```python
from build123d import *

# Parameters (mm, degrees)
F0_W         = 50.8
F0_H         = 25.4
F0_R         = 3.3655
F1_DEPTH     = 17.78
F2_W         = 9.906
F2_H         = 25.4
F3_DEPTH     = 9.906
F5_DEPTH     = 2.54
F6_R         = 5.08
F7_T1_DEPTH  = 25.4
F7_T3_DEPTH  = 4.826
F7_T5_DEPTH  = 15.24
F7_T7_DEPTH  = 2.286
F7_T10_ANGLE = 90
F7_T12_ANGLE = 90
F7_T14_ANGLE = 90
F7_T16_ANGLE = 90
F7_T18_ANGLE = 90
F7_T20_ANGLE = 90
F7_T22_ANGLE = 90
F7_T24_ANGLE = 90


# Not quite as in the source:
# - a fillet or chamfer that OpenCascade refuses, or shapes differently, is made with other operations: its cross-section is extruded or revolved along the edge and cut away or added
# - a feature names something its author has since deleted; it is built from what else it names


with BuildPart() as f1:
    # F0 (on Top) → F1 (new body)
    with BuildSketch(Plane.XY):
        with Locations((20.1624472324, -3.7984256737)):
            Rectangle(F0_W, F0_H)
        with Locations((7.4624472324, -3.7984256737)):
            Circle(F0_R, mode=Mode.SUBTRACT)
        with Locations((32.8624472324, -3.7984256737)):
            Circle(F0_R, mode=Mode.SUBTRACT)
    extrude(amount=F1_DEPTH)

    # F2 (on face) → F3 (cut)
    with BuildSketch(Plane.XY.offset(17.78)):
        with Locations((20.5434472324, -3.7984256737)):
            Rectangle(F2_W, F2_H)
    extrude(amount=-F3_DEPTH, mode=Mode.SUBTRACT)

    # F4 (on face) → F5 (cut)
    with BuildSketch(Plane.XY.offset(17.78)):
        Polygon((29.6874472324, -9.2976869878), (36.0374472324, -9.2976869878), (39.2124472324, -3.7984256737), (36.0374472324, 1.7008356403), (29.6874472324, 1.7008356403), (26.5124472324, -3.7984256737), align=None)
        Polygon((4.2874472324, -9.2976869878), (10.6374472324, -9.2976869878), (13.8124472324, -3.7984256737), (10.6374472324, 1.7008356403), (4.2874472324, 1.7008356403), (1.1124472324, -3.7984256737), align=None)
    extrude(amount=-F5_DEPTH, mode=Mode.SUBTRACT)

    # F6
    f6_edges = [f1.edges().sort_by_distance(p)[0] for p in [
        (45.562447, -3.798426, 17.78),
        (5.176447, 8.901574, 17.78),
        (-5.237553, -3.798426, 17.78),
        (5.176447, -16.498426, 17.78),
        (35.529447, -16.498426, 17.78),
        (35.529447, 8.901574, 17.78),
        (-5.237553, 8.901574, 8.89),
        (-5.237553, -16.498426, 8.89),
        (45.562447, -16.498426, 8.89),
        (45.562447, 8.901574, 8.89),
    ]]
    fillet(f6_edges, radius=F6_R)

    # F7: fillet of radius 2.54 on 10 edges, made by hand

    # F7_s2 → F7_t1 (join)
    with BuildSketch(Plane.XZ.offset(-8.9015743263)):
        with BuildLine():
            ThreePointArc((15.5904472324, 10.414), (16.3343960082, 8.6179487758), (18.1304472324, 7.874))
            Line((18.1304472324, 7.874), (15.5904472324, 7.874))
            Line((15.5904472324, 7.874), (15.5904472324, 10.414))
        make_face()
        with BuildLine():
            ThreePointArc((25.4964472324, 10.414), (24.7524984566, 8.6179487758), (22.9564472324, 7.874))
            Line((22.9564472324, 7.874), (25.4964472324, 7.874))
            Line((25.4964472324, 7.874), (25.4964472324, 10.414))
        make_face()
    extrude(amount=F7_T1_DEPTH)

    # F7_s4 → F7_t3 (cut)
    with BuildSketch(Plane.YZ.offset(18.1304472324)):
        with BuildLine():
            ThreePointArc((6.3615743263, 7.874), (8.1576255505, 7.1300512242), (8.9015743263, 5.334))
            Line((8.9015743263, 5.334), (8.9015743263, 7.874))
            Line((8.9015743263, 7.874), (6.3615743263, 7.874))
        make_face()
        with BuildLine():
            ThreePointArc((-16.4984256737, 5.334), (-15.7544768979, 7.1300512242), (-13.9584256737, 7.874))
            Line((-13.9584256737, 7.874), (-16.4984256737, 7.874))
            Line((-16.4984256737, 7.874), (-16.4984256737, 5.334))
        make_face()
    extrude(amount=F7_T3_DEPTH, mode=Mode.SUBTRACT)

    # F7_s6 → F7_t5 (cut)
    with BuildSketch(Plane.XZ.offset(-3.8215743263)):
        with BuildLine():
            ThreePointArc((15.5904472324, 15.24), (14.8464984566, 17.0360512242), (13.0504472324, 17.78))
            Line((13.0504472324, 17.78), (15.5904472324, 17.78))
            Line((15.5904472324, 17.78), (15.5904472324, 15.24))
        make_face()
        with BuildLine():
            ThreePointArc((25.4964472324, 15.24), (26.2403960082, 17.0360512242), (28.0364472324, 17.78))
            Line((28.0364472324, 17.78), (25.4964472324, 17.78))
            Line((25.4964472324, 17.78), (25.4964472324, 15.24))
        make_face()
    extrude(amount=F7_T5_DEPTH, mode=Mode.SUBTRACT)

    # F7_s8 → F7_t7 (cut)
    with BuildSketch(Plane.XY.offset(10.414)):
        with BuildLine():
            ThreePointArc((25.4964472324, 6.3615743263), (26.2403960082, 8.1576255505), (28.0364472324, 8.9015743263))
            Line((28.0364472324, 8.9015743263), (25.4964472324, 8.9015743263))
            Line((25.4964472324, 8.9015743263), (25.4964472324, 6.3615743263))
        make_face()
        with BuildLine():
            ThreePointArc((15.5904472324, 6.3615743263), (14.8464984566, 8.1576255505), (13.0504472324, 8.9015743263))
            Line((13.0504472324, 8.9015743263), (15.5904472324, 8.9015743263))
            Line((15.5904472324, 8.9015743263), (15.5904472324, 6.3615743263))
        make_face()
        with BuildLine():
            ThreePointArc((28.0364472324, -16.4984256737), (26.2403960082, -15.7544768979), (25.4964472324, -13.9584256737))
            Line((25.4964472324, -13.9584256737), (25.4964472324, -16.4984256737))
            Line((25.4964472324, -16.4984256737), (28.0364472324, -16.4984256737))
        make_face()
        with BuildLine():
            ThreePointArc((13.0504472324, -16.4984256737), (14.8464984566, -15.7544768979), (15.5904472324, -13.9584256737))
            Line((15.5904472324, -13.9584256737), (15.5904472324, -16.4984256737))
            Line((15.5904472324, -16.4984256737), (13.0504472324, -16.4984256737))
        make_face()
    extrude(amount=F7_T7_DEPTH, mode=Mode.SUBTRACT)

    # F7_s9 → F7_t10 (revolve, cut)
    with BuildSketch(Plane.XY.offset(12.7)):
        with BuildLine():
            ThreePointArc((13.0504472324, -16.4984256737), (14.8464984566, -15.7544768979), (15.5904472324, -13.9584256737))
            Line((15.5904472324, -13.9584256737), (15.5904472324, -16.4984256737))
            Line((15.5904472324, -16.4984256737), (13.0504472324, -16.4984256737))
        make_face()
    revolve(axis=Axis((15.5904472324, -11.4184256737, 12.7), (-1, 0, 0)), revolution_arc=F7_T10_ANGLE, mode=Mode.SUBTRACT)

    # F7_s11 → F7_t12 (revolve, cut)
    with BuildSketch(Plane.XY.offset(12.7)):
        with BuildLine():
            ThreePointArc((28.0364472324, -16.4984256737), (26.2403960082, -15.7544768979), (25.4964472324, -13.9584256737))
            Line((25.4964472324, -13.9584256737), (25.4964472324, -16.4984256737))
            Line((25.4964472324, -16.4984256737), (28.0364472324, -16.4984256737))
        make_face()
    revolve(axis=Axis((25.4964472324, -11.4184256737, 12.7), (-1, 0, 0)), revolution_arc=F7_T12_ANGLE, mode=Mode.SUBTRACT)

    # F7_s13 → F7_t14 (revolve, cut)
    with BuildSketch(Plane.XZ.offset(-3.8215743263)):
        with BuildLine():
            ThreePointArc((15.5904472324, 15.24), (14.8464984566, 17.0360512242), (13.0504472324, 17.78))
            Line((13.0504472324, 17.78), (15.5904472324, 17.78))
            Line((15.5904472324, 17.78), (15.5904472324, 15.24))
        make_face()
    revolve(axis=Axis((15.5904472324, 3.8215743263, 12.7), (-1, 0, 0)), revolution_arc=F7_T14_ANGLE, mode=Mode.SUBTRACT)

    # F7_s15 → F7_t16 (revolve, cut)
    with BuildSketch(Plane.XZ.offset(-3.8215743263)):
        with BuildLine():
            ThreePointArc((25.4964472324, 15.24), (26.2403960082, 17.0360512242), (28.0364472324, 17.78))
            Line((28.0364472324, 17.78), (25.4964472324, 17.78))
            Line((25.4964472324, 17.78), (25.4964472324, 15.24))
        make_face()
    revolve(axis=Axis((25.4964472324, 3.8215743263, 12.7), (-1, 0, 0)), revolution_arc=F7_T16_ANGLE, mode=Mode.SUBTRACT)

    # F7_s17 → F7_t18 (revolve, cut)
    with BuildSketch(Plane.XY.offset(10.414)):
        with BuildLine():
            ThreePointArc((13.0504472324, -16.4984256737), (14.8464984566, -15.7544768979), (15.5904472324, -13.9584256737))
            Line((15.5904472324, -13.9584256737), (15.5904472324, -16.4984256737))
            Line((15.5904472324, -16.4984256737), (13.0504472324, -16.4984256737))
        make_face()
    revolve(axis=Axis((18.1304472324, -16.4984256737, 10.414), (0, -1, 0)), revolution_arc=F7_T18_ANGLE, mode=Mode.SUBTRACT)

    # F7_s19 → F7_t20 (revolve, cut)
    with BuildSketch(Plane.XY.offset(10.414)):
        with BuildLine():
            ThreePointArc((28.0364472324, -16.4984256737), (26.2403960082, -15.7544768979), (25.4964472324, -13.9584256737))
            Line((25.4964472324, -13.9584256737), (25.4964472324, -16.4984256737))
            Line((25.4964472324, -16.4984256737), (28.0364472324, -16.4984256737))
        make_face()
    revolve(axis=Axis((22.9564472324, -16.4984256737, 10.414), (0, 1, 0)), revolution_arc=F7_T20_ANGLE, mode=Mode.SUBTRACT)

    # F7_s21 → F7_t22 (revolve, cut)
    with BuildSketch(Plane.XY.offset(10.414)):
        with BuildLine():
            ThreePointArc((13.0504472324, 8.9015743263), (14.8464984566, 8.1576255505), (15.5904472324, 6.3615743263))
            Line((15.5904472324, 6.3615743263), (15.5904472324, 8.9015743263))
            Line((15.5904472324, 8.9015743263), (13.0504472324, 8.9015743263))
        make_face()
    revolve(axis=Axis((18.1304472324, 8.9015743263, 10.414), (0, -1, 0)), revolution_arc=F7_T22_ANGLE, mode=Mode.SUBTRACT)

    # F7_s23 → F7_t24 (revolve, cut)
    with BuildSketch(Plane.XY.offset(10.414)):
        with BuildLine():
            ThreePointArc((28.0364472324, 8.9015743263), (26.2403960082, 8.1576255505), (25.4964472324, 6.3615743263))
            Line((25.4964472324, 6.3615743263), (25.4964472324, 8.9015743263))
            Line((25.4964472324, 8.9015743263), (28.0364472324, 8.9015743263))
        make_face()
    revolve(axis=Axis((22.9564472324, 8.9015743263, 10.414), (0, 1, 0)), revolution_arc=F7_T24_ANGLE, mode=Mode.SUBTRACT)


solid = f1.part
```
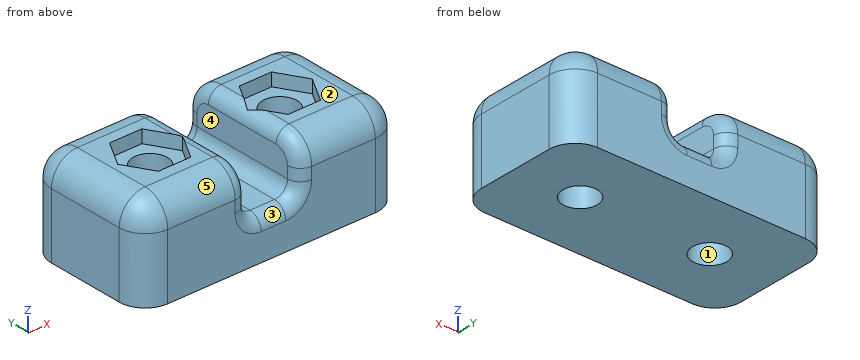
Check sheet for the modelled part. Datum: model origin and axes. Units: mm. Face numbers are marked on the shaded views. A direction names the side the tool comes from. Coordinates: 2 decimals unless noted, no trailing zeros. Order: outer loops, then holes, each group sorted by start corner. A loop starts at its lowest first (then second) coordinate and runs counter-clockwise, first axis right, second up. Notation, with made-up numbers: (33.5, 54.25) -> (74.5, 54.25) arc R11 ccw to (74.5, 59.25) -> close; hole circle Ø8 at (-26, 30.25). An arc over 180 degrees is marked (long way). Write each question's results on one line, items separated by ' | '. Start each with the question number.
1) Set-up check for the marked faces 4 and 5: record each of +Z, -Z, +X, -X, +Y, -Y from which the full face is reachable in a straight line by a thin tool's end or side.
2) Section check A-A (z = 11). Enter the section's corners in (x, y).
3) Section check C-C (x = 33). Enter the section's corners in (y, z).
4) Draft check along Y on the marked faces 1, 2 and 3. Enter one of: pulls with the +Y half, pulls with the -Y half, needs draft (parallel to the pull), parting line crosses it, or undercut.
5) Section check B-B (z = 3). Enter the section's corners in (x, y).
6) Depth check by flat-ended pin: pin 1 (1.3 mm diameter, centred on x = 34, z = 16.5, fed in from +Y); pin 2 (3 mm diameter, centred on x = 6.5, z = 16.5, fed in from -Y); pin 3 (5.5 mm diameter, centred on x = 9, y = -5.5, fed in from +Z). Enter the tip coordinate at first touch or a pass-through.
7) Section check D-D (y = 1). Enter the section's corners in (x, z), and give its area (3 significant figures).
8) Material ranges on line 1 along X through (y, z) = (-9.5, 11.75); line 2 along Z through (x, y) = (13, -3.5); line 3 along Y through (x, z) = (10.5, 3), recorded low to high.
Checked values:
1) face 4: +Z, +Y, -Y | face 5: +Z, +X, -X, -Y
2) outline: (-5.24, -11.42) arc R5.08 ccw to (-0.16, -16.5) -> (13.05, -16.5) arc R2.54 ccw to (15.59, -13.96) -> (15.59, 6.36) arc R2.54 ccw to (13.05, 8.9) -> (-0.16, 8.9) arc R5.08 ccw to (-5.24, 3.82) -> close; (25.5, -13.96) arc R2.54 ccw to (28.04, -16.5) -> (40.48, -16.5) arc R5.08 ccw to (45.56, -11.42) -> (45.56, 3.82) arc R5.08 ccw to (40.48, 8.9) -> (28.04, 8.9) arc R2.54 ccw to (25.5, 6.36) -> close; hole circle Ø6.73 at (7.46, -3.8); hole circle Ø6.73 at (32.86, -3.8)
3) outline: (-16.5, 0) -> (-7.16, 0) -> (-7.16, 15.24) -> (-9.3, 15.24) -> (-9.3, 17.78) -> (-11.42, 17.78) arc R5.08 ccw to (-16.5, 12.7) -> close; (-0.44, 0) -> (8.9, 0) -> (8.9, 12.7) arc R5.08 ccw to (3.82, 17.78) -> (1.7, 17.78) -> (1.7, 15.24) -> (-0.44, 15.24) -> close
4) face 1: undercut | face 2: needs draft | face 3: pulls with the -Y half
5) outline: (-5.24, -11.42) arc R5.08 ccw to (-0.16, -16.5) -> (40.48, -16.5) arc R5.08 ccw to (45.56, -11.42) -> (45.56, 3.82) arc R5.08 ccw to (40.48, 8.9) -> (-0.16, 8.9) arc R5.08 ccw to (-5.24, 3.82) -> close; hole circle Ø6.73 at (7.46, -3.8); hole circle Ø6.73 at (32.86, -3.8)
6) pin 1: y = 7.81 | pin 2: y = -15.95 | pin 3: z = 15.24
7) outline: (-5.24, 0) -> (45.56, 0) -> (45.56, 12.7) arc R5.08 ccw to (40.48, 17.78) -> (36.44, 17.78) -> (36.44, 15.24) -> (29.28, 15.24) -> (29.28, 17.78) -> (28.04, 17.78) arc R2.54 ccw to (25.5, 15.24) -> (25.5, 10.41) arc R2.54 cw to (22.96, 7.87) -> (18.13, 7.87) arc R2.54 cw to (15.59, 10.41) -> (15.59, 15.24) arc R2.54 ccw to (13.05, 17.78) -> (11.04, 17.78) -> (11.04, 15.24) -> (3.88, 15.24) -> (3.88, 17.78) -> (-0.16, 17.78) arc R5.08 ccw to (-5.24, 12.7) -> close | area: 758 mm²
8) line 1: -5.24 to 15.59, 25.5 to 45.56 | line 2: 0 to 15.24 | line 3: -16.5 to -5.25, -2.35 to 8.9
